```python
from build123d import *

# Parameters (mm, degrees)
SKETCH1_W           = 20.06486665
SKETCH1_H           = 63.9
SKETCH1_R           = 3.35
BOSS_EXTRUDE1_DEPTH = 6.5
CHAMFER1_SIZE       = 1


with BuildPart() as part:
    # Sketch1 → Boss-Extrude1 (new body)
    with BuildSketch(Plane(origin=(0, 0, 0), x_dir=(1, 0, 0), z_dir=(0, 1, 0))):
        with Locations((-10.582433325, -32.5)):
            Rectangle(SKETCH1_W, SKETCH1_H)
        with Locations((-10.582433325, -15.25)):
            Circle(SKETCH1_R, mode=Mode.SUBTRACT)
        with Locations((-10.582433325, -49.75)):
            Circle(SKETCH1_R, mode=Mode.SUBTRACT)
    extrude(amount=BOSS_EXTRUDE1_DEPTH)

    # Chamfer1
    chamfer1_edges = [part.edges().sort_by_distance(p)[0] for p in [
        (-13.932433325, 6.5, 15.25),
        (-13.932433325, 6.5, 49.75),
    ]]
    chamfer(chamfer1_edges, length=CHAMFER1_SIZE)


solid = part.part
```
CAD build for the part. Positions are in the model's coordinates, mm. Round coordinates to 2 decimals unless told otherwise and drop trailing zeros. Order: outer loops, then holes, each group sorted by start corner. A loop starts at its lowest first (then second) coordinate and runs counter-clockwise, first axis right, second up.
Q1. Two-plate mould, pull along X, no slides. Class faces 1 (the cylindrical face through (-13.052, 2.712, 12.986)), 2 (the flat face through (-11, 3, 0.55)), 3 (the flat face through (-20.615, 3, 33)): pulls with the +X half, pulls with the -X half, needs draft (parallel to the pull), parting line crosses it, or undercut.
Q2. Slice it at B-B (y = 3). Write the cut outline in (x, z).
Q3. Wall check: L1, parallel to X at y = 2.25, z = 49.75; L2, parallel to Z at x = -13, y = 3.5; L3, parallel to Z at x = -10, y = 2.5. Give the ranges that are in metal, low to high.
Q4. Drop a flat-ended pin along its axis: pin 1 (3 mm diameter, centred on x = -7, z = 37, fed in from -Y). Give the stop position or say it passes through.
Q5. Slice it at C-C (x = -10.5). State how many separate pieces and enclosed holes the cut face has, and give its area (3 significant figures).
Q6. Slice it at A-A (z = 49.75). Write the cut outline in (x, y).
Results below:
1. face 1: undercut
1. face 2: needs draft
1. face 3: pulls with the -X half
2. outline: (-20.61, 0.55) - (-0.55, 0.55) - (-0.55, 64.45) - (-20.61, 64.45) - close; hole circle Ø6.7 at (-10.58, 15.25); hole circle Ø6.7 at (-10.58, 49.75)
3. L1: x = -20.61 to -13.93, -7.23 to -0.55
3. L2: z = 0.55 to 12.93, 17.57 to 47.43, 52.07 to 64.45
3. L3: z = 0.55 to 11.95, 18.55 to 46.45, 53.05 to 64.45
4. pin 1: stops at y = 0
5. separate pieces: 3
5. enclosed holes: 0
5. area: 326 mm2
6. outline: (-20.61, 0) - (-13.93, 0) - (-13.93, 5.5) - (-14.93, 6.5) - (-20.61, 6.5) - close; (-7.23, 0) - (-0.55, 0) - (-0.55, 6.5) - (-6.23, 6.5) - (-7.23, 5.5) - close
